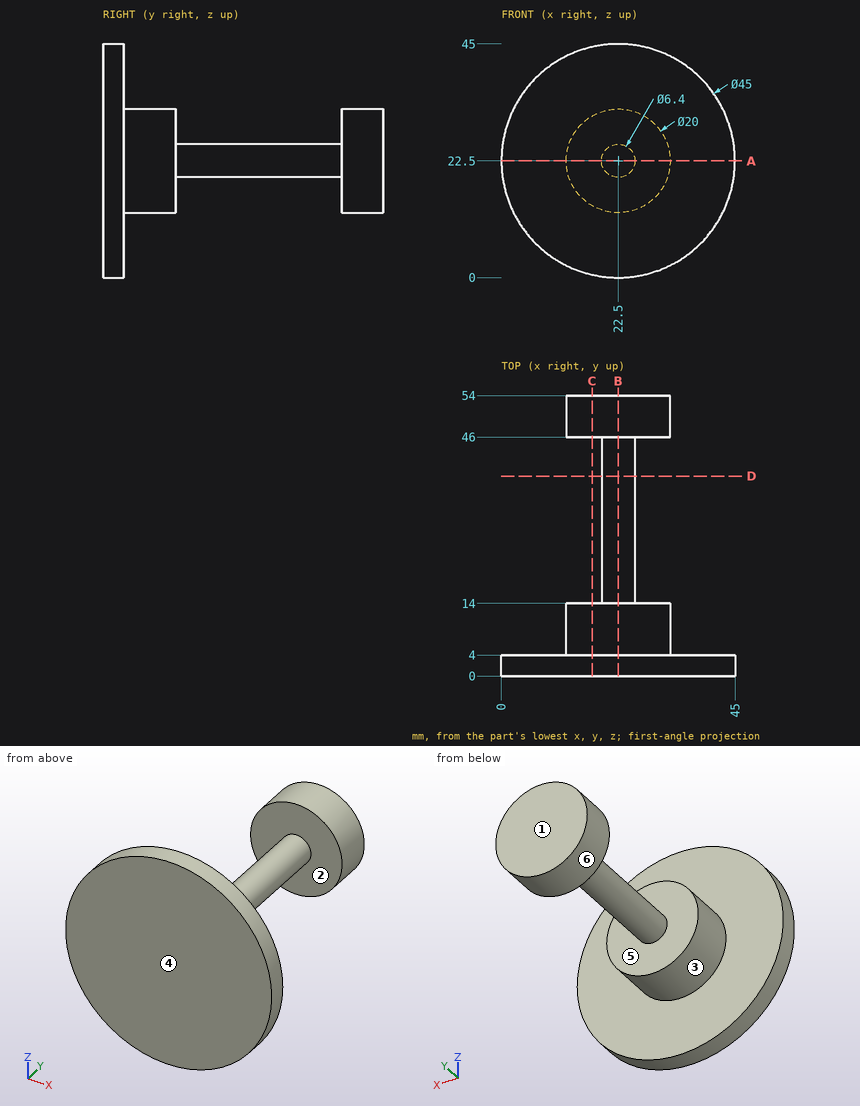
Here's the drawing with two shaded views (mm, measured from the low corner). I have some questions. A direction names the side the tool comes from. Give positions to 0.01 mm unless a question says otherwise; leave off trailing zeros. Write each loop counter-clockwise with the first axis right and the second up, starting at its lowest first coordinate (ties: lowest second). Pieces come first, ordered by that corner, then holes. Notation, with made-up numbers: (70, -35.75) -> (117, -35.75) arc R16 ccw to (117, -5.75) -> close; hole circle Ø7 at (10.25, -31). An arc over 180 degrees is marked (long way). Use one line per item in the form item = value. Start each with the question number.
1. Imagine slicing it at D-D on y = 38.5. List the corners of the cut face in (x, z) for me.
2. Imagine slicing it at B-B on x = 22.5. List the corners of the cut face in (y, z) for me, plus the area to 3 significant figures.
3. Will these pins go through, and if not, where does the flat tip stop? pin 1 Ø3 at (y, z) = (43, 21) entering from +X; pin 2 Ø10 at (x, z) = (30.5, 34) entering from +Y; pin 3 Ø8 at (x, y) = (20, 11.5) entering from -Z; pin 4 Ø4 at (y, z) = (12, 28) entering from -X.
4. On a 3-axis mill with a long thin cutter (end or side, diameter ignored), from which of +Z, -Z, +X, -X, +Y, -Y can I reach the whole of each face in a straight line? I mean the marked faces 4, 5 and 6. Say none if no direction works.
5. If I drill on L1, parallel to Y at x = 23, z = 16; L2, parallel to X at y = 47.5, z = 22; L3, parallel to Y at x = 10.5, z = 8, over which ranges is the centre line in solid material (lowest first)?
6. Thinking about a two-plate mould opening in Y: for the marked faces 1, 2 and 3, which applies, +Y half, -Y half, draft (parallel to the pull), parting line (faces both ways), or undercut?
7. Imagine slicing it at A-A on z = 22.5. List the corners of the cut face in (x, y) for me, plus the area to 3 significant figures.
8. Imagine slicing it at C-C on x = 17.5. List the corners of the cut face in (y, z) for me, plus the area to 3 significant figures.
Entries:
q1.outline = circle Ø6.4 at (22.5, 22.5)
q2.outline = (0, 0) -> (4, 0) -> (4, 12.5) -> (14, 12.5) -> (14, 19.3) -> (46, 19.3) -> (46, 12.5) -> (54, 12.5) -> (54, 32.5) -> (46, 32.5) -> (46, 25.7) -> (14, 25.7) -> (14, 32.5) -> (4, 32.5) -> (4, 45) -> (0, 45) -> close
q2.area = 745 mm²
q3.pin_1 = 25.7
q3.pin_2 = 54
q3.pin_3 = 12.5
q3.pin_4 = 13.13
q4.face_4 = +Z, -Z, +X, -X, -Y
q4.face_5 = none
q4.face_6 = +Y
q5.L1 = 0 to 14, 46 to 54
q5.L2 = 12.51 to 32.49
q5.L3 = 0 to 4
q6.face_1 = +Y half
q6.face_2 = undercut
q6.face_3 = draft
q7.outline = (0, 0) -> (45, 0) -> (45, 4) -> (32.5, 4) -> (32.5, 14) -> (25.7, 14) -> (25.7, 46) -> (32.5, 46) -> (32.5, 54) -> (12.5, 54) -> (12.5, 46) -> (19.3, 46) -> (19.3, 14) -> (12.5, 14) -> (12.5, 4) -> (0, 4) -> close
q7.area = 745 mm²
q8.outline = (0, 0.56) -> (4, 0.56) -> (4, 13.84) -> (14, 13.84) -> (14, 31.16) -> (4, 31.16) -> (4, 44.44) -> (0, 44.44) -> close; (46, 13.84) -> (54, 13.84) -> (54, 31.16) -> (46, 31.16) -> close
q8.area = 487 mm²
